from build123d import *

# Parameters (mm, degrees)
SKETCH1_W           = 93
SKETCH1_H           = 49
BOSS_EXTRUDE1_DEPTH = 2.6
SKETCH2_W           = 10
SKETCH2_H           = 2.5
CUT_EXTRUDE1_DEPTH  = 2.6
BOSS_EXTRUDE2_DEPTH = 2.6


with BuildPart() as part:
    # Sketch1 → Boss-Extrude1 (new body)
    with BuildSketch(Plane(origin=(0, 0, 0), x_dir=(1, 0, 0), z_dir=(0, 1, 0))):
        Rectangle(SKETCH1_W, SKETCH1_H)
    extrude(amount=BOSS_EXTRUDE1_DEPTH)

    # Sketch2 → Cut-Extrude1 (cut)
    with BuildSketch(Plane(origin=(0, 2.6, 0), x_dir=(1, 0, 0), z_dir=(0, 1, 0))):
        with Locations((0, 23.25)):
            Rectangle(SKETCH2_W, SKETCH2_H)
    extrude(amount=-CUT_EXTRUDE1_DEPTH, mode=Mode.SUBTRACT)

    # Sketch3 → Boss-Extrude2 (add)
    with BuildSketch(Plane.XZ):
        Polygon((-16.5, 23), (-16.5, 26), (-10.5, 26), (-10.5, 23), (-10.5, 21.5), (-16.5, 21.5), align=None)
        Polygon((10.5, 23), (10.5, 26), (16.5, 26), (16.5, 23), (16.5, 21.5), (10.5, 21.5), align=None)
    extrude(amount=BOSS_EXTRUDE2_DEPTH)


solid = part.part
CAD build for the part. Positions are in the model's coordinates, mm. A direction names the side the tool comes from. Round coordinates to 2 decimals unless told otherwise and drop trailing zeros. Order: outer loops, then holes, each group sorted by start corner. A loop starts at its lowest first (then second) coordinate and runs counter-clockwise, first axis right, second up. Notation, with made-up numbers: (-4.5, 24) -> (31.5, 24) arc R13 cw to (31.5, 28) -> close; hole circle Ø4 at (-9.75, -1). An arc over 180 degrees is marked (long way). Write item = value, one per line. Start each with the question number.
(1) Cut at A-A, the plane y = 1.05. List the corners of the cut face in (x, z).
(2) Probe line 1 (Z direction, x = 6.5, y = 1.6); line 2 (Y direction, x = -14.5, z = -12); line 3 (Z direction, x = 4.5, y = 2.1). List the from-to ranges inside material, lowest first. Write a range as [from, to].
(3) Pull direction X, two halves, no side cores. Call faces 1 (the flat face through (13, -1, 26)), 2 (the flat face through (-5, 1, -23)), 3 (the flat face through (46.5, 1, 0)): released by +X, released by -X, zero draft, split by the parting line, or undercut.
(4) Cut at B-B, the plane z = 5. List the corners of the cut face in (x, y), then the cut area to 3 significant figures.
(5) Pin check, flat tips, straight feed: P1, Ø12, axis at x = -21.5, z = -3, coming from the -Y side; P2, Ø1.3, axis at x = 8.5, y = 1, coming from the +Z side; P3, Ø0.8, axis at x = 13, z = 25.5, coming from the +Y side; P4, Ø1, axis at y = -1, z = 8.5, coming from the +X side. Stop position of each tip, or through.
(6) Which spindle directions (+Z, -Z, +X, -X, +Y, -Y) get a long thin tool onto all of the face, cutting with end or side? Do faces 4 (the flat face through (10.5, -1, 24)), 5 (the flat face through (-16.5, -1, 24)), 6 (the flat face through (0, 1, -22)), 7 (the flat face through (-13, -1, 21.5)). Say none if no direction does.
(7) Cut at C-C, the plane x = -19. List the corners of the cut face in (y, z), then the cut area to 3 significant figures.
Model answer:
q1.outline = (-46.5, -24.5) -> (-5, -24.5) -> (-5, -22) -> (5, -22) -> (5, -24.5) -> (46.5, -24.5) -> (46.5, 24.5) -> (-46.5, 24.5) -> close
q2.line_1 = [-24.5, 24.5]
q2.line_2 = [0, 2.6]
q2.line_3 = [-22, 24.5]
q3.face_1 = zero draft
q3.face_2 = undercut
q3.face_3 = released by +X
q4.outline = (-46.5, 0) -> (46.5, 0) -> (46.5, 2.6) -> (-46.5, 2.6) -> close
q4.area = 242 mm2
q5.P1 = 0
q5.P2 = 24.5
q5.P3 = 0
q5.P4 = through
q6.face_4 = +Z, -Z, -Y
q6.face_5 = +Z, -Z, -X, -Y
q6.face_6 = -Z, +Y, -Y
q6.face_7 = -Z, +X, -X, -Y
q7.outline = (0, -24.5) -> (2.6, -24.5) -> (2.6, 24.5) -> (0, 24.5) -> close
q7.area = 127 mm2
